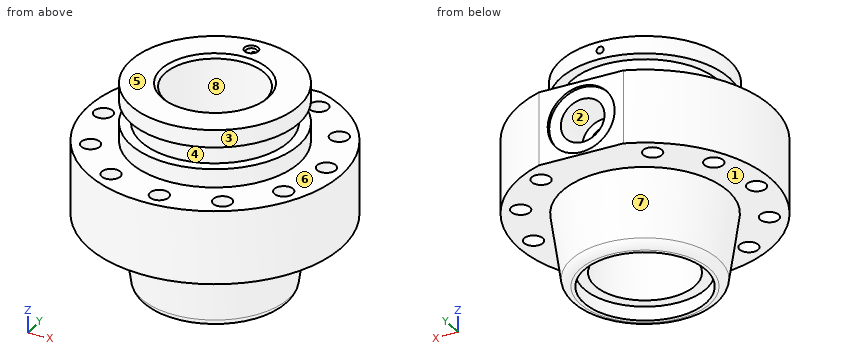
from build123d import *

# Parameters (mm, degrees)
SKETCH1_R               = 72.5
BOSS_EXTRUDE1_DEPTH     = 42
SKETCH2_R               = 48.2
BOSS_EXTRUDE2_DEPTH     = 33
SKETCH4_R               = 28.6
CUT_EXTRUDE1_DEPTH      = 156.568312969
SKETCH5_R               = 35
CUT_EXTRUDE2_DEPTH      = 8
SKETCH6_W               = 12.5
SKETCH6_H               = 6
FILLET1_R               = 5
SKETCH7_R               = 5.35
CUT_EXTRUDE3_DEPTH      = 133.546218354
CIRPATTERN1_COUNT       = 12
CHAMFER1_SIZE           = 2
SKETCH8_W               = 51
SKETCH8_H               = 57.058415431
CUT_EXTRUDE4_DEPTH      = 22
CUT_EXTRUDE4_DEPTH_BACK = 1.6
SKETCH9_R               = 19
CUT_EXTRUDE5_DEPTH      = 1.6
SKETCH10_R              = 5.35
BOSS_EXTRUDE3_DEPTH     = 42
SKETCH11_R              = 12.4
CUT_EXTRUDE6_DEPTH      = 23
SKETCH12_R              = 19
CUT_EXTRUDE7_DEPTH      = 23
SKETCH13_R              = 7.5
CUT_EXTRUDE8_DEPTH      = 23
CUT_EXTRUDE9_REACH      = 157.568
CUT_EXTRUDE9_END_RADIUS = 7.5
SKETCH14_R              = 3
CHAMFER2_SIZE           = 1
CUT_EXTRUDE10_START     = 40
SKETCH15_R              = 2
CUT_EXTRUDE10_DEPTH     = 88.033460159


with BuildPart() as part:
    # Sketch1 → Boss-Extrude1 (new body)
    with BuildSketch(Plane.XY):
        with Locations(Location((0, 0, 0), (0, 0, 180))):
            Circle(SKETCH1_R)
    extrude(amount=BOSS_EXTRUDE1_DEPTH)

    # Sketch2 → Boss-Extrude2 (add)
    with BuildSketch(Plane.XY.offset(42)):
        Circle(SKETCH2_R)
    extrude(amount=BOSS_EXTRUDE2_DEPTH)

    # Sketch3 → Revolve1 (revolve)
    with BuildSketch(Plane(origin=(0, 0, 0), x_dir=(0, 0, -1), z_dir=(1, 0, 0)), mode=Mode.PRIVATE) as revolve1_sk:
        Polygon((0, 47.6), (42, 41.5), (42, 28.6), (0, 28.6), align=None)
    revolve(revolve1_sk.sketch.rotate(Axis((0, 0, 0), (0, 0, -1)), 90), axis=Axis((0, 0, 0), (0, 0, -1)))

    # Sketch4 → Cut-Extrude1 (cut, through all)
    with BuildSketch(Plane.XY.offset(75)):
        Circle(SKETCH4_R)
    extrude(amount=-CUT_EXTRUDE1_DEPTH, mode=Mode.SUBTRACT)

    # Sketch5 → Cut-Extrude2 (cut)
    with BuildSketch(Plane(origin=(0, 0, -42), x_dir=(-1, 0, 0), z_dir=(0, 0, -1))):
        Circle(SKETCH5_R)
    extrude(amount=-CUT_EXTRUDE2_DEPTH, mode=Mode.SUBTRACT)

    # Sketch6 → Cut-Revolve1 (revolve, cut)
    with BuildSketch(Plane(origin=(0, 0, 0), x_dir=(0, 0, -1), z_dir=(1, 0, 0)), mode=Mode.PRIVATE) as cut_revolve1_sk:
        with Locations((-58.75, 45.2)):
            Rectangle(SKETCH6_W, SKETCH6_H)
    revolve(cut_revolve1_sk.sketch.rotate(Axis((0, 0, 75), (0, 0, -1)), 90), axis=Axis((0, 0, 75), (0, 0, -1)), mode=Mode.SUBTRACT)

    # Fillet1
    fillet1_edges = [part.edges().sort_by_distance(p)[0] for p in [
        (-41.5, 0, -42),
    ]]
    fillet(fillet1_edges, radius=FILLET1_R)

    # Sketch7 → Cut-Extrude3 (cut, through all)
    with BuildSketch(Plane.XY.offset(42)):
        with Locations((-1.544322391, 62.480917634)):
            Circle(SKETCH7_R)
    cut_extrude3 = extrude(amount=-CUT_EXTRUDE3_DEPTH, mode=Mode.SUBTRACT)

    # CirPattern1: Cut-Extrude3 ×12 about axis
    cirpattern1_axis = Axis((0, 0, 0), (0, 0, 1))
    for i in range(1, CIRPATTERN1_COUNT):
        add(cut_extrude3.rotate(cirpattern1_axis, i * 360 / CIRPATTERN1_COUNT), mode=Mode.SUBTRACT)

    # Chamfer1
    chamfer1_edges = [part.edges().sort_by_distance(p)[0] for p in [
        (-28.6, 0, 75),
    ]]
    chamfer(chamfer1_edges, length=CHAMFER1_SIZE)

    # Sketch8 → Cut-Extrude4 (cut, two sides)
    with BuildSketch(Plane(origin=(0, 70, 0), x_dir=(1, 0, 0), z_dir=(0, 1, 0))) as cut_extrude4_sk:
        with Locations((0, -20.682853763)):
            Rectangle(SKETCH8_W, SKETCH8_H)
    extrude(amount=CUT_EXTRUDE4_DEPTH, mode=Mode.SUBTRACT)
    extrude(cut_extrude4_sk.sketch, amount=-CUT_EXTRUDE4_DEPTH_BACK, mode=Mode.SUBTRACT)

    # Sketch9 → Cut-Extrude5 (cut)
    with BuildSketch(Plane(origin=(0, 68.4, 0), x_dir=(1, 0, 0), z_dir=(0, 1, 0))):
        with Locations(Location((0, -20.30259433, 0), (0, 0, 270))):
            Circle(SKETCH9_R)
    extrude(amount=-CUT_EXTRUDE5_DEPTH, mode=Mode.SUBTRACT)

    # Sketch10 → Boss-Extrude3 (add)
    with BuildSketch(Plane.XY.offset(42)):
        with Locations((-1.544322391, 62.480917634)):
            Circle(SKETCH10_R)
    extrude(amount=-BOSS_EXTRUDE3_DEPTH)

    # Sketch11 → Cut-Extrude6 (cut)
    with BuildSketch(Plane(origin=(0, 66.8, 0), x_dir=(1, 0, 0), z_dir=(0, 1, 0))):
        with Locations(Location((0, -20.30259433, 0), (0, 0, 270))):
            Circle(SKETCH11_R)
    extrude(amount=-CUT_EXTRUDE6_DEPTH, mode=Mode.SUBTRACT)

    # Sketch12 → Cut-Extrude7 (cut)
    with BuildSketch(Plane(origin=(0, 66.8, 0), x_dir=(1, 0, 0), z_dir=(0, 1, 0))):
        with Locations(Location((0, -20.30259433, 0), (0, 0, 270))):
            Circle(SKETCH12_R)
    extrude(amount=CUT_EXTRUDE7_DEPTH, mode=Mode.SUBTRACT)

    # Sketch13 → Cut-Extrude8 (cut)
    with BuildSketch(Plane(origin=(0, 43.8, 0), x_dir=(1, 0, 0), z_dir=(0, 1, 0))):
        with Locations(Location((0, -20.30259433, 0), (0, 0, 270))):
            Circle(SKETCH13_R)
    extrude(amount=-CUT_EXTRUDE8_DEPTH, mode=Mode.SUBTRACT)

    # Cut-Extrude9: up to this cylinder (the profile starts outside it)
    cut_extrude9_end = Plane(origin=(0, 39, 20.30259433), z_dir=(0, 1, 0)) * Cylinder(CUT_EXTRUDE9_END_RADIUS, 331.136, mode=Mode.PRIVATE)
    # Sketch14 → Cut-Extrude9 (cut, up to the surface)
    with BuildSketch(Plane.XY.offset(75), mode=Mode.PRIVATE) as cut_extrude9_sk1:
        with Locations((0, 39)):
            Circle(SKETCH14_R)
    cut_extrude9_tool1 = extrude(cut_extrude9_sk1.sketch, amount=-CUT_EXTRUDE9_REACH, mode=Mode.PRIVATE) - cut_extrude9_end
    add(cut_extrude9_tool1.solids().sort_by_distance((0, 39, 75))[0], mode=Mode.SUBTRACT)

    # Chamfer2
    chamfer2_edges = [part.edges().sort_by_distance(p)[0] for p in [
        (-3, 39, 75),
    ]]
    chamfer(chamfer2_edges, length=CHAMFER2_SIZE)

    # Sketch15 → Cut-Extrude10 (cut, through all)
    with BuildSketch(Plane(origin=(0, 0, 0), x_dir=(1, 0, 0), z_dir=(0, 1, 0)).offset(CUT_EXTRUDE10_START)):
        with Locations(Location((0, -70, 0), (0, 0, 90))):
            Circle(SKETCH15_R)
    extrude(amount=CUT_EXTRUDE10_DEPTH, mode=Mode.SUBTRACT)


solid = part.part
Check sheet for the modelled part. Datum: model origin and axes. Units: mm. Face numbers are marked on the shaded views. A direction names the side the tool comes from. Round coordinates to 2 decimals unless told otherwise and drop trailing zeros. Write each loop counter-clockwise with the first axis right and the second up, starting at its lowest first coordinate (ties: lowest second). Pieces come first, ordered by that corner, then holes. Notation, with made-up numbers: (56.5, 37) - (60.5, 37) arc R25 ccw to (60.5, 75) - close; hole circle Ø5 at (41, 29). An arc over 180 degrees is marked (long way). Return JSON: item names as keys, results as strings.
Q1. Depth check by flat-ended pin: P1, Ø3, axis at x = -20, y = -49, coming from the +Z side; P2, Ø17, axis at x = 0, z = 20.3, coming from the -Y side; P3, Ø12.5, axis at x = -29.9, y = -54.88, coming from the -Z side; P4, Ø8, axis at x = 0, y = 39, coming from the -Z side. Enter the tip coordinate at first touch or a pass-through.
Returned:
{"P1": "stops at z = 42", "P2": "stops at y = -72.5", "P3": "stops at z = 0", "P4": "stops at z = -42"}
Q2. Cross-section at B-B (z = 47). Record the boundary of the cut face in (x, y), then the cut area to 3 significant figures.
Returned:
{"outline": "circle Ø96.4 at (0, 0); hole circle Ø57.2 at (0, 0); hole circle Ø6 at (0, 39)", "area": "4,700 mm²"}
Q3. Draft check along Y on the marked faces 6, 7 and 8. Enter one of: released by +Y, released by -Y, zero draft, split by the parting line, or undercut.
Returned:
{"face 6": "zero draft", "face 7": "split by the parting line", "face 8": "undercut"}
Q4. Access from +Z, -Z, +X, -X, +Y, -Y to the whole of each face (thin tool, end or side, straight path). Record for the marked faces 1, 2, 3, 4 and 5.
Returned:
{"face 1": "-Z", "face 2": "+Y", "face 3": "+Z", "face 4": "none", "face 5": "+Z, +X, -X, +Y, -Y"}
Q5. Cross-section at A-A (z = 17). Give the number of separate pieces and of enclosed holes in the cut face, then the cut area to 3 significant figures.
Returned:
{"separate pieces": "1", "enclosed holes": "11", "area": "12,000 mm²"}
Q6. Scan lines: L1, parallel to Y at x = 0, z = 43; L2, parallel to Y at x = -0.5, z = 34; L3, parallel to Y at x = 0, z = -38.25. Record each from-to range of solid material in increasing order. Write a range as from..to.
Returned:
{"L1": "y = -48.2..-28.6, 28.6..36, 42..48.2", "L2": "y = -72.5..-67.42, -57.54..-28.6, 28.6..36.04, 41.96..66.8", "L3": "y = -42.01..-35, 35..42.01"}
Q7. Cross-section at C-C (z = 70). Record the boundary of the cut face in (x, y), then the cut area to 4 significant figures.
Returned:
{"outline": "(-2, 41.24) - (-2, 48.16) arc R48.2 ccw (long way) to (2, 48.16) - (2, 41.24) arc R3 cw (long way) to start; hole circle Ø57.2 at (0, 0)", "area": "4,675 mm²"}
